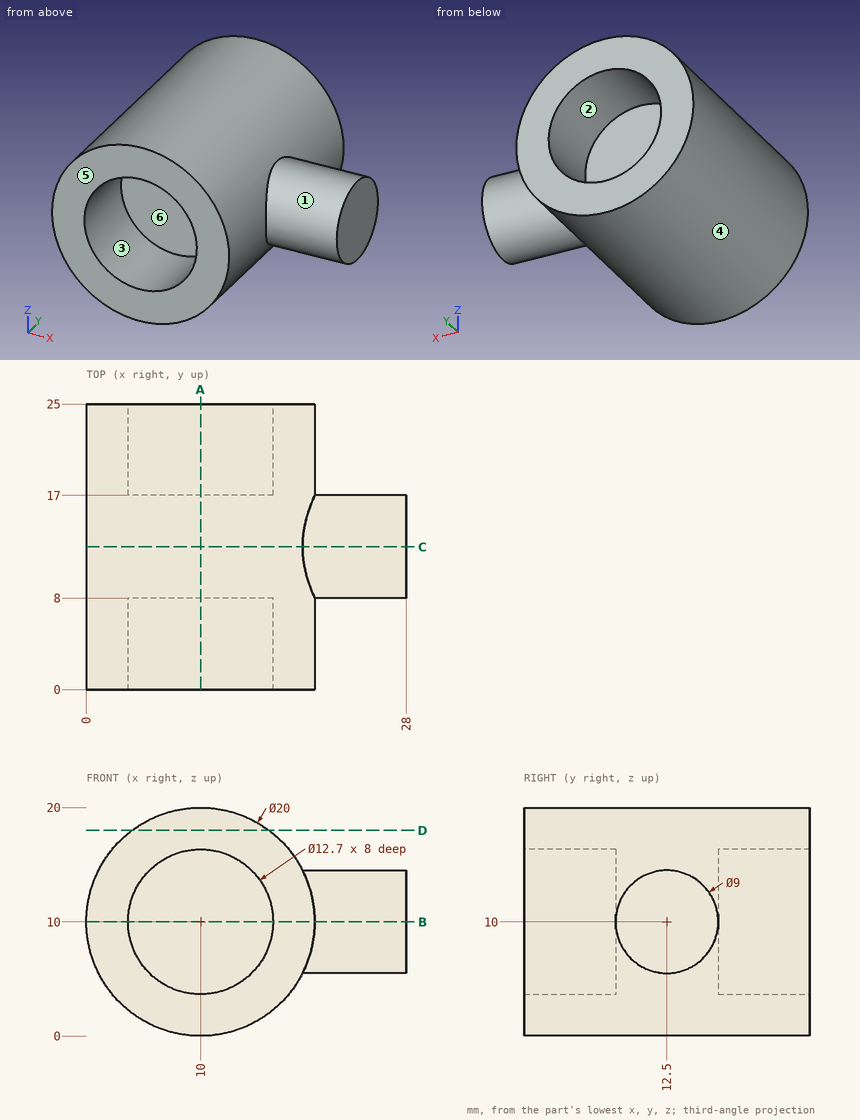
Drawing for the job (mm, zero at the part's lowest x, y, z). A direction names the side the tool comes from. Round coordinates to 2 decimals unless told otherwise and drop trailing zeros. Loops run counter-clockwise (first coordinate to the right, second up) from the corner with the lowest first, then second, coordinate; pieces in that order, holes last.
1. Drop flat-ended pins along their axis: P1, Ø3, axis at y = 9.5, z = 13.5, coming from the -X side; P2, Ø12, axis at y = 14.5, z = 15.5, coming from the +X side; P3, Ø6.5, axis at x = 8.5, z = 12.5, coming from the +Y side; P4, Ø3, axis at x = 13, z = 8, coming from the -Y side. Give the stop position or say it passes through.
Check values:
P1: stops at x = 0.2
P2: stops at x = 28
P3: stops at y = 17
P4: stops at y = 8
2. Mould opens along Z. For the marked faces 4, 5 and 6 say: +Z half, -Z half, draft (parallel to the pull), parting line (faces both ways), or undercut.
Check values:
face 4: parting line
face 5: draft
face 6: undercut
3. Band-saw the part on A-A, the plane x = 10. List the corners of the cut face in (y, z), and give its area (3 significant figures).
Check values:
outline: (0, 0) - (25, 0) - (25, 3.65) - (17, 3.65) - (17, 16.35) - (25, 16.35) - (25, 20) - (0, 20) - (0, 16.35) - (8, 16.35) - (8, 3.65) - (0, 3.65) - close
area: 297 mm2
4. Band-saw the part on B-B, the plane z = 10. List the corners of the cut face in (x, y).
Check values:
outline: (0, 0) - (3.65, 0) - (3.65, 8) - (16.35, 8) - (16.35, 0) - (20, 0) - (20, 8) - (28, 8) - (28, 17) - (20, 17) - (20, 25) - (16.35, 25) - (16.35, 17) - (3.65, 17) - (3.65, 25) - (0, 25) - close
5. Band-saw the part on C-C, the plane y = 12.5. List the corners of the cut face in (x, z).
Check values:
outline: (18.93, 5.5) - (28, 5.5) - (28, 14.5) - (18.93, 14.5) arc R10 ccw (long way) to start
6. Band-saw the part on D-D, the plane z = 18. List the corners of the cut face in (x, y), and give its area (3 significant figures).
Check values:
outline: (4, 0) - (16, 0) - (16, 25) - (4, 25) - close
area: 300 mm2
7. Tool access for the marked faces 1, 2 and 3: list every direction of +Z, -Z, +X, -X, +Y, -Y with a clear straight run to the whole face (end or side of a thin tool).
Check values:
face 1: +X
face 2: +Y
face 3: -Y
8. Wall check: probe 1 along Y at (x, z) = (11.25, 7); probe 2 along X at (y, z) = (4.75, 10); probe 3 along X at (y, z) = (3.75, 6.75). Give the ranges that are in metal, low to high.
Check values:
probe 1: y = 8 to 17
probe 2: x = 0 to 3.65, 16.35 to 20
probe 3: x = 0.54 to 4.54, 15.46 to 19.46
